```python
from build123d import *

# Parameters (mm, degrees)
EXTRUDE_1_DEPTH = 2
SKETCH_3_R      = 0.5
EXTRUDE_3_DEPTH = 52
SKETCH_4_R      = 0.5
EXTRUDE_4_DEPTH = 58


with BuildPart() as part:
    # Эскиз1 → Бобышка-Вытянуть1 (new body)
    with BuildSketch(Plane(origin=(0, 0, 0), x_dir=(0, 0, -1), z_dir=(1, 0, 0))):
        Polygon((-26, 6.284861441), (-23.051215157, 5.974931665), (-14.51812841, 0), (0, 0), (0, 58), (-20.56451991, 58), align=None)
    extrude(amount=EXTRUDE_1_DEPTH)

    # Эскиз3 → Бобышка-Вытянуть3 (add)
    with BuildSketch(Plane(origin=(0, 3.513339809, -0.369266894), x_dir=(1, 0, 0), z_dir=(0, -0.9945218953682733, 0.10452846326765391))):
        with BuildLine():
            Line((0, 26.514516188), (0, 27.514516188))
            ThreePointArc((0, 27.514516188), (1, 28.514516188), (2, 27.514516188))
            Line((2, 27.514516188), (2, 26.514516188))
            Line((2, 26.514516188), (0, 26.514516188))
        make_face()
        with Locations(Location((1, 27.514516188, 0), (0, 0, 270))):
            Circle(SKETCH_3_R, mode=Mode.SUBTRACT)
    extrude(amount=-EXTRUDE_3_DEPTH)

    # Эскиз4 → Бобышка-Вытянуть4 (add)
    with BuildSketch(Plane(origin=(0, 0, 0), x_dir=(1, 0, 0), z_dir=(0, 1, 0))):
        with BuildLine():
            Line((-1, 0), (0, 0))
            Line((0, 0), (0, -2))
            Line((0, -2), (-1, -2))
            ThreePointArc((-1, -2), (-2, -1), (-1, 0))
        make_face()
        with Locations(Location((-1, -1, 0), (0, 0, 90))):
            Circle(SKETCH_4_R, mode=Mode.SUBTRACT)
    extrude(amount=EXTRUDE_4_DEPTH)


solid = part.part
```
Geometry: final body of the model. Coordinates: model frame, mm. A direction names the side the tool comes from. Round coordinates to 2 decimals unless told otherwise and drop trailing zeros. Write each loop counter-clockwise with the first axis right and the second up, starting at its lowest first coordinate (ties: lowest second). Pieces come first, ordered by that corner, then holes. Notation, with made-up numbers: (-22, 55) -> (-13, 55) arc R19 ccw to (-13, 88) -> close; hole circle Ø3 at (14, 1). An arc over 180 degrees is marked (long way). Use CSV: the item, a comma, the result in double quotes. Start each with the question number.
Q1. Section A-A (y = 36.5). Give the number of separate pieces and of enclosed holes in the cut face, plus the area to 3 significant figures.
Q2. Reachability of faces 1 (the face through (1, 0, 7)), 2 (the face through (-0.5, 28.6, 2)) from +Z, -Z, +X, -X, +Y, -Y: full face, straight path, thin tool, end or side. Return the list, or none.
Q3. Pull-direction query (X, two-part tool) for faces 3 (the face through (-0.7, 28.6, 1.4)), 4 (the face through (-2, 29, 1)), 5 (the face through (1, 58, 10)); classes: pulls with the +X half, pulls with the -X half, needs draft (parallel to the pull), parting line crosses it, or undercut.
Q4. Line query: L1, parallel to X at y = 19, z = 1; L2, parallel to X at y = 16, z = 5.25; L3, parallel to Y at x = 0.25, z = 1.25. Output: solid intervals per line, ascending.
Q5. Section B-B (z = 17.25). Return loops of the section in (x, y), plus the area to 3 significant figures.
Q6. First-contact query: pin 1 Ø12.5 at (y, z) = (25.5, 12.5) entering from -X; pin 2 Ø1 at (x, y) = (-1.5, 21) entering from +Z; pin 3 Ø2 at (x, z) = (1.5, 18) entering from -Y. Flat tips, straight axial feed; report the tip coordinate or a pass-through.
Result sheet:
1,separate pieces,"1"
1,enclosed holes,"2"
1,area,"51.2 mm²"
2,face 1,"+Z, -Z, +X, -X, -Y"
2,face 2,"+Z, -X, +Y, -Y"
3,face 3,"undercut"
3,face 4,"pulls with the -X half"
3,face 5,"needs draft"
4,L1,"-2 to -1.5, -0.5 to 2"
4,L2,"0 to 2"
4,L3,"0 to 58"
5,outline,"(0, 1.91) -> (2, 1.91) -> (2, 58) -> (0, 58) -> close"
5,area,"112 mm²"
6,pin 1,"x = 0"
6,pin 2,"z = 2"
6,pin 3,"y = 1.74"
